The model under review builds one solid part; all positions refer to its coordinate system, in mm. Face numbers are marked on the shaded views. Coordinates: 2 decimals unless noted, no trailing zeros. Order: outer loops, then holes, each group sorted by start corner. A loop starts at its lowest first (then second) coordinate and runs counter-clockwise, first axis right, second up. Notation, with made-up numbers: M -36.75,12 L -23.75,12 A12 cw -23.75,26 Z; hole C 65.5,20 d9. An arc over 180 degrees is marked long. Answer in a Markdown table with one row per item.
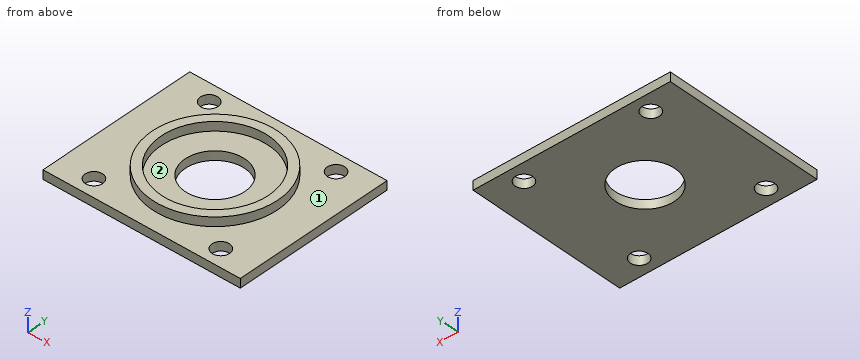
Autodesk Inventor part; units mm, degrees
ref_plane "YZ Plane" through (0, 0, 0) normal (1, 0, 0) x (0, 1, 0)
ref_plane "XZ Plane" through (0, 0, 0) normal (0, 1, 0) x (-1, 0, 0)
ref_plane "XY Plane" through (0, 0, 0) normal (0, 0, 1) x (1, 0, 0)
sketch "Sketch1" plane through (0, 0, 0) normal (0, 0, 1) x (1, 0, 0)
  line L0 (0, 0) -> (-69.85, 0)
  line L1 (-69.85, 0) -> (-69.85, 57.15)
  line L2 (-69.85, 57.15) -> (0, 57.15)
  line L3 (0, 57.15) -> (0, 0)
  dimension "d0" = 69.85
  dimension "d1" = 57.15
extrude "Extrusion1" add sketch "Sketch1" along normal blind 3.175
sketch "Sketch2" plane through (0, 0, 3.175) normal (0, 0, 1) x (1, 0, 0)
  line L0 (-69.85, 57.15) -> (-69.85, 0) construction
  line L1 (-69.85, 0) -> (0, 0) construction
  line L2 (-69.85, 57.15) -> (0, 0) construction
  circle A0 centre (-34.925, 28.575) radius 22.225
  dimension "d4" = 44.45
extrude "Extrusion2" add sketch "Sketch2" along normal blind 3.175
sketch "Sketch3" plane through (0, 0, 3.175) normal (0, 0, 1) x (1, 0, 0)
  circle A0 centre (-34.925, 28.575) radius 22.225 construction
  circle A1 centre (-34.925, 28.575) radius 31.75 construction
  line L0 (-34.925, 28.575) -> (-12.4744, 6.1244) construction
  line L1 (-34.925, 28.575) -> (-3.175, 28.575) construction
  circle A2 centre (-12.4744, 6.1244) radius 3.1
  circle A3 centre (-12.4744, 51.0256) radius 3.1
  circle A4 centre (-57.3756, 51.0256) radius 3.1
  circle A5 centre (-57.3756, 6.1244) radius 3.1
  point P0 (0, 0)
  dimension "d7" = 63.5
  dimension "d8" = 45
  dimension "d9" = 6.2
  dimension "d12" = 360
extrude "Extrusion3" cut sketch "Sketch3" against normal blind 3.175
sketch "Sketch4" plane through (-34.925, 28.575, 6.35) normal (0, 0, 1) x (1, 0, 0)
  circle A0 centre (0, 0) radius 19.05
  point P0 (34.925, -28.575)
  dimension "d16" = 38.1
extrude "Extrusion4" cut sketch "Sketch4" against normal blind 3.175
sketch "Sketch5" plane through (-34.925, 28.575, 3.175) normal (0, 0, 1) x (1, 0, 0)
  circle A0 centre (0, 0) radius 10.541
  point P0 (34.925, -28.575)
  dimension "d19" = 21.082
extrude "Extrusion5" cut sketch "Sketch5" against normal blind 3.175
properties part number "endcap2" material "Aluminum 6061"
(1) Insertion check: P1, Ø1.5, axis at x = -20.5, y = 10, coming from the +Z side (3 decimals); P2, Ø1, axis at x = -18, z = 5.5, coming from the +Y side. Each pin has a flat end and moves straight along its axis. Give the tip position at first contact, or say it passes through.
Report:
| item | result |
|---|---|
| P1 | z = 3.175 |
| P2 | y = 43.55 |
(2) Take a section at A-A (y = 37). Write out the cut boundary in (x, z) (3 decimals).
Report:
| item | result |
|---|---|
| outline | M -69.85,0 L -41.26,0 L -41.26,3.175 L -52.011,3.175 L -52.011,6.35 L -55.491,6.35 L -55.491,3.175 L -69.85,3.175 Z; M -28.59,0 L 0,0 L 0,3.175 L -14.359,3.175 L -14.359,6.35 L -17.839,6.35 L -17.839,3.175 L -28.59,3.175 Z |
(3) To check wall thickness, follow line 1 (X direction, y = 4, z = 0.75); line 2 (Z direction, x = -22.5, y = 49.5) (3 decimals); line 3 (X direction, y = 30.5, z = 0.75). State the ranges of each line that lie inside material, in increasing order. Write a range as [from, to].
Report:
| item | result |
|---|---|
| line 1 | [-69.85, -59.63], [-55.12, -14.73], [-10.22, 0] |
| line 2 | [0, 3.175] |
| line 3 | [-69.85, -45.29], [-24.56, 0] |
(4) Take a section at B-B (x = -32). Write out the cut boundary in (y, z) (3 decimals).
Report:
| item | result |
|---|---|
| outline | M 0,0 L 18.448,0 L 18.448,3.175 L 9.751,3.175 L 9.751,6.35 L 6.543,6.35 L 6.543,3.175 L 0,3.175 Z; M 38.702,0 L 57.15,0 L 57.15,3.175 L 50.607,3.175 L 50.607,6.35 L 47.399,6.35 L 47.399,3.175 L 38.702,3.175 Z |
(5) Take a section at C-C (z = 2). Write out the cut boundary in (x, y) (3 decimals).
Report:
| item | result |
|---|---|
| outline | M -69.85,0 L 0,0 L 0,57.15 L -69.85,57.15 Z; hole C -57.376,6.124 d6.2; hole C -57.376,51.026 d6.2; hole C -34.925,28.575 d21.082; hole C -12.474,6.124 d6.2; hole C -12.474,51.026 d6.2 |
(6) The part is to be moulded in two halves that separate along X. For the marked faces 1 and 2, say which applies: +X half, -X half, draft (parallel to the pull), parting line (faces both ways), or undercut.
Report:
| item | result |
|---|---|
| face 1 | draft |
| face 2 | undercut |
(7) Take a section at D-D (y = 5). State how many separate pieces and enclosed holes the cut face has, then the cut area to 3 significant figures.
Report:
| item | result |
|---|---|
| separate pieces | 3 |
| enclosed holes | 0 |
| area | 185 mm^2 |
